from build123d import *

# Parameters (mm, degrees)
EXTRUDE_1_DEPTH     = 17
SKETCH_2_W          = 17
SKETCH_2_H          = 13
CUT_EXTRUDE_1_DEPTH = 18
CUT_EXTRUDE_2_DEPTH = 4


with BuildPart() as part:
    # 草图1 → 凸台-拉伸1 (new body)
    with BuildSketch(Plane.XY):
        Polygon((0, 0), (20, 0), (20, 3), (3, 20), (0, 20), align=None)
    extrude(amount=EXTRUDE_1_DEPTH)

    # 草图2 → 切除-拉伸1 (cut, through all)
    with BuildSketch(Plane(origin=(0, 3, 0), x_dir=(-1, 0, 0), z_dir=(0, -1, 0))):
        with Locations((-11.5, -8.5)):
            Rectangle(SKETCH_2_W, SKETCH_2_H)
    extrude(amount=-CUT_EXTRUDE_1_DEPTH, mode=Mode.SUBTRACT)

    # 草图5 → 切除-拉伸2 (cut, through all)
    with BuildSketch(Plane(origin=(0, 3, 0), x_dir=(1, 0, 0), z_dir=(0, 1, 0))):
        with BuildLine():
            Line((11.75, -11.45), (8.85, -11.45))
            ThreePointArc((8.85, -11.45), (5.9, -8.5), (8.85, -5.55))
            Line((8.85, -5.55), (11.75, -5.55))
            ThreePointArc((11.75, -5.55), (14.7, -8.5), (11.75, -11.45))
        make_face()
    cut_extrude_2 = extrude(amount=-CUT_EXTRUDE_2_DEPTH, mode=Mode.SUBTRACT)

    # 镜向1: 切除-拉伸2 across plane
    add(cut_extrude_2.mirror(Plane(origin=(0, 0, 0), x_dir=(0, 0, 1), z_dir=(0.707106781, -0.707106781, 0))), mode=Mode.SUBTRACT)


solid = part.part
Here's how the part is built. I have some questions about the finished solid (model axes, mm). A direction names the side the tool comes from. Coordinates: 2 decimals unless noted, no trailing zeros. Order: outer loops, then holes, each group sorted by start corner. A loop starts at its lowest first (then second) coordinate and runs counter-clockwise, first axis right, second up.
Item 1: If we section it at B-B on y = 7.75: List the corners of the cut face in (x, z) for me, plus the area to 3 significant figures.
Result sheet:
outline: (0, 0) - (15.25, 0) - (15.25, 2) - (3, 2) - (3, 5.76) - (0, 5.76) - close; (0, 11.24) - (3, 11.24) - (3, 15) - (15.25, 15) - (15.25, 17) - (0, 17) - close
area: 83.6 mm2
Item 2: For faces 4 (the face through (14, 3, 6)), 5 (the face through (2, 20, 8)), 6 (the face through (10, 2, 5.55)), 7 (the face through (8, 8, 0)), 8 (the face through (1.5, 14.7, 8.4)), which set-ups out of +Z, -Z, +X, -X, +Y, -Y let a thin tool reach every point of the face, with its end or its side?
Result sheet:
face 4: +X, +Y
face 5: +Z, -Z, +X, -X, +Y
face 6: +Y, -Y
face 7: -Z, +X, -X, +Y, -Y
face 8: +X, -X
Item 3: For P1, Ø4, axis at y = 14, z = 15, coming from the +X side; P2, Ø5, axis at x = 11, z = 10, coming from the +Y side; P3, Ø4, axis at y = 7.5, z = 9, coming from the +X side, each with a flat end and sliding along its axis, tell me the tip position at first contact or that it passes through.
Result sheet:
P1: stops at x = 11
P2: stops at y = 3
P3: stops at x = 3
Item 4: I need wall thicknesses on line 1 (Z direction, x = 6.5, y = 16.25); line 2 (X direction, y = 3.75, z = 12.5); line 3 (Z direction, x = 2.5, y = 7). Which ranges of each line are inside material? Lowest first, please.
Result sheet:
line 1: z = 0 to 2, 15 to 17
line 2: x = 0 to 3
line 3: z = 0 to 6.2, 10.8 to 17
Item 5: If we section it at C-C on y = 18.25: List the corners of the cut face in (x, z) for me, plus the area to 3 significant figures.
Result sheet:
outline: (0, 0) - (4.75, 0) - (4.75, 2) - (3, 2) - (3, 15) - (4.75, 15) - (4.75, 17) - (0, 17) - close
area: 58.0 mm2
Item 6: If we section it at D-D on x = 18.5: List the corners of the cut face in (y, z) for me, plus the area to 3 significant figures.
Result sheet:
outline: (0, 0) - (4.5, 0) - (4.5, 2) - (3, 2) - (3, 15) - (4.5, 15) - (4.5, 17) - (0, 17) - close
area: 57.0 mm2
Item 7: If we section it at A-A on z = 8.5: List the corners of the cut face in (x, y) for me.
Result sheet:
outline: (0, 0) - (5.9, 0) - (5.9, 3) - (3, 3) - (3, 5.9) - (0, 5.9) - close; (0, 14.7) - (3, 14.7) - (3, 20) - (0, 20) - close; (14.7, 0) - (20, 0) - (20, 3) - (14.7, 3) - close
Item 8: If we mould it in two halves opening along X, with no side actions, what happens to faces 1 (the face through (3, 13.3, 11.5)), 2 (the face through (0, 10, 5)), 3 (the face through (10, 2, 11.45))? For each: +X half, -X half, draft (parallel to the pull), parting line (faces both ways), or undercut.
Result sheet:
face 1: +X half
face 2: -X half
face 3: undercut
